Here's the drawing with two shaded views (mm, measured from the low corner). I have some questions. A direction names the side the tool comes from. Coordinates: 2 decimals unless noted, no trailing zeros. Write each loop counter-clockwise with the first axis right and the second up, starting at its lowest first coordinate (ties: lowest second). Pieces come first, ordered by that corner, then holes. Notation, with made-up numbers: (15, 26) - (30, 26) arc R29 cw to (30, 59) - close; hole circle Ø5 at (32, 43.5). An arc over 180 degrees is marked (long way). Answer in a Markdown table with one row per item. Add a question column.
Item 1: Imagine slicing it at C-C (y = 23). Please give me the cut outline in (x, z).
Item 2: I'm going to push flat-ended pins straight in: pin 1 (2 mm diameter, centred on y = 83.5, z = 25.5, fed in from +X); pin 2 (5 mm diameter, centred on x = 61.5, y = 57, fed in from +Z); pin 3 (6 mm diameter, centred on x = 20.5, y = 70, fed in from -Z) (1 decimal). Where does each tip first touch, or does it pass through?
Item 3: Imagine slicing it at D-D (z = 113). Please give me the cut outline in (x, y), plus the area to 3 significant figures.
Item 4: We'd pull the mould along Y, two halves only. Please class the marked faces 1, 2, 3 and 4: +Y half, -Y half, draft (parallel to the pull), parting line (faces both ways), or undercut.
Item 5: Imagine slicing it at A-A (z = 22). Please give me the cut outline in (x, y), plus the area to 3 significant figures.
Item 6: If I drill on probe 1 along X at (y, z) = (68.5, 75); probe 2 along Y at (x, z) = (45.5, 63); probe 3 along X at (y, z) = (31.5, 60), over which ranges is the centre line in solid material (lowest first)? Write a range as from..to.
Item 7: Imagine slicing it at B-B (x = 6.5). Please give me the cut outline in (y, z) (1 decimal), plus the area to 3 significant figures.
Item 8: Which directions (+Z, -Z, +X, -X, +Y, -Y) give clear straight access to the entire face, cutting with the end or side of a thin tool? Please do the marked faces 5 and 6.
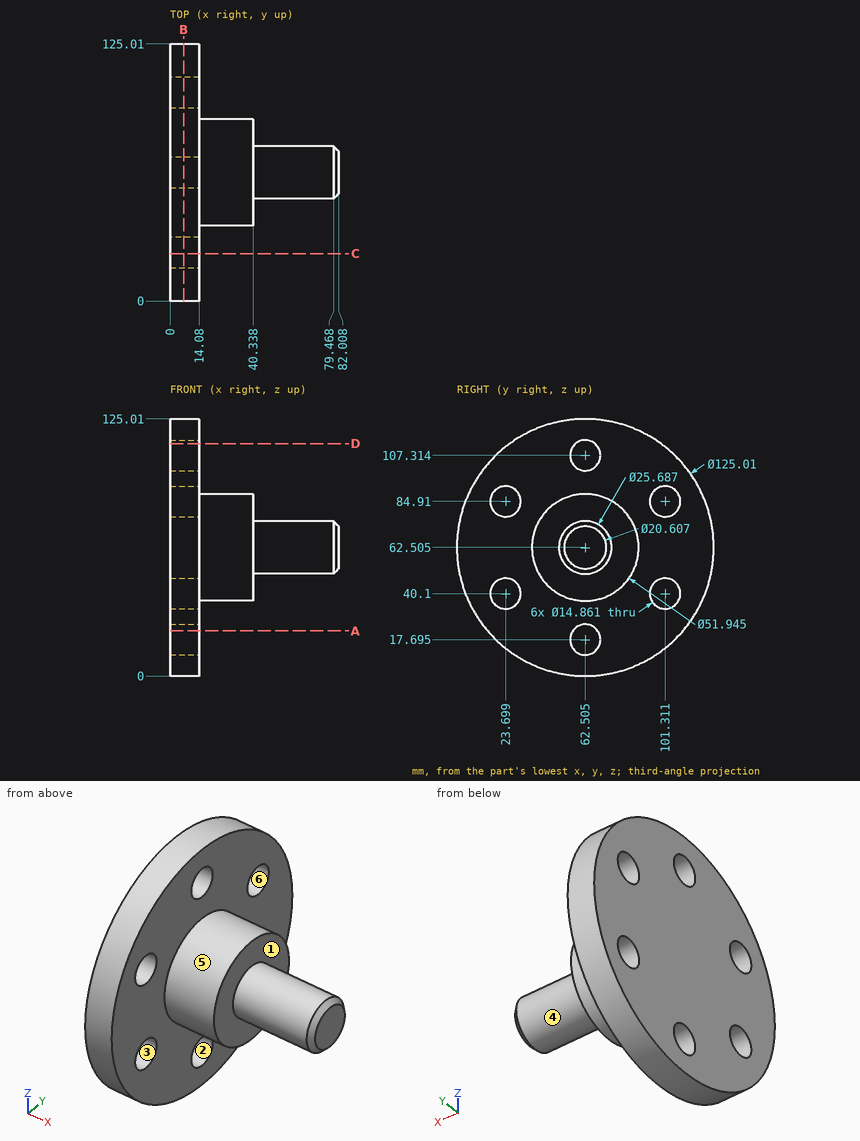
Here are the results:
| question | item | result |
|---|---|---|
| 1 | outline | (0, 14.07) - (14.08, 14.07) - (14.08, 32.7) - (0, 32.7) - close; (0, 47.5) - (14.08, 47.5) - (14.08, 77.51) - (0, 77.51) - close; (0, 92.31) - (14.08, 92.31) - (14.08, 110.94) - (0, 110.94) - close |
| 2 | pin 1 | stops at x = 14.08 |
| 2 | pin 2 | stops at z = 74.99 |
| 2 | pin 3 | stops at z = 36.9 |
| 3 | outline | (0, 25.67) - (14.08, 25.67) - (14.08, 57.72) - (0, 57.72) - close; (0, 67.29) - (14.08, 67.29) - (14.08, 99.34) - (0, 99.34) - close |
| 3 | area | 903 mm2 |
| 4 | face 1 | draft |
| 4 | face 2 | undercut |
| 4 | face 3 | undercut |
| 4 | face 4 | parting line |
| 5 | outline | (0, 14.9) - (14.08, 14.9) - (14.08, 56.45) - (0, 56.45) - close; (0, 68.56) - (14.08, 68.56) - (14.08, 110.11) - (0, 110.11) - close |
| 5 | area | 1,170 mm2 |
| 6 | probe 1 | x = 0..40.34 |
| 6 | probe 2 | y = 49.67..75.34 |
| 6 | probe 3 | x = 0..14.08 |
| 7 | outline | circle Ø125 at (62.5, 62.5); hole circle Ø14.9 at (23.7, 40.1); hole circle Ø14.9 at (23.7, 84.9); hole circle Ø14.9 at (62.5, 17.7); hole circle Ø14.9 at (62.5, 107.3); hole circle Ø14.9 at (101.3, 40.1); hole circle Ø14.9 at (101.3, 84.9) |
| 7 | area | 11,200 mm2 |
| 8 | face 5 | +X |
| 8 | face 6 | +X, -X |
